Autodesk Inventor part; units mm, degrees
ref_plane "YZ Plane" through (0, 0, 0) normal (1, 0, 0) x (0, 1, 0)
ref_plane "XZ Plane" through (0, 0, 0) normal (0, 1, 0) x (-1, 0, 0)
ref_plane "XY Plane" through (0, 0, 0) normal (0, 0, 1) x (1, 0, 0)
sketch "Sketch1" plane through (0, 0, 0) normal (1, 0, 0) x (0, 1, 0)
  line L0 (15, 25) -> (-5, 25)
  line L1 (-5, 25) -> (-5, -25)
  line L2 (-5, -25) -> (15, -25)
  line L3 (15, -25) -> (0, -10)
  line L4 (0, -10) -> (0, 10)
  line L5 (0, 10) -> (15, 25)
  line L6 (0, 0) -> (-5, 0) construction
  circle A0 centre (5, -20) radius 2
  circle A1 centre (5, 20) radius 2
  dimension "d0" = 50
  dimension "d1" = 45
  dimension "d2" = 5
  dimension "d4" = 40
  dimension "d5" = 4
  dimension "d6" = 20
  dimension "d7" = 5
  dimension "d8" = 15
extrude "Extrusion1" add sketch "Sketch1" along normal blind 5
sketch "Sketch2" plane through (0, 0, 0) normal (-1, 0, 0) x (0, 0, 1)
  line L0 (25, -5) -> (-25, -5)
  line L1 (-25, -5) -> (25, -5)
  line L2 (25, -5) -> (25, 0)
  line L3 (25, 0) -> (-25, 0)
  line L4 (-25, 0) -> (-25, -5)
  point P0 (0, 0)
extrude "Extrusion2" add sketch "Sketch2" along normal blind 10
mirror "Mirror1" about plane through (-10, -2.5, 0) normal (-1, 0, 0)
sketch "Sketch5" plane through (5, -5, -25) normal (0, -1, 0) x (1, 0, 0)
  line L0 (0, 50) -> (0, 0) construction
  line L1 (0, 50) -> (-30, 50)
  line L2 (-30, 50) -> (-30, 55)
  line L3 (-30, 55) -> (0, 55)
  line L4 (0, 55) -> (0, 50)
  line L5 (-30, 0) -> (0, 0)
  line L6 (0, 0) -> (-30, 0)
  line L7 (-30, 0) -> (-30, -5)
  line L8 (-30, -5) -> (0, -5)
  line L9 (0, -5) -> (0, 0)
  line L10 (-30, 50) -> (-30, 0) construction
  point P0 (-5, 25)
  dimension "d19" = 5
extrude "Extrusion5" add sketch "Sketch5" against normal blind 62.5
sketch "Sketch6" plane through (-25, -5, 30) normal (0, 0, 1) x (1, 0, 0)
  line L0 (30, 62.5) -> (25, 62.5)
  line L1 (25, 62.5) -> (25, 47.5)
  line L2 (25, 47.5) -> (30, 47.5)
  line L3 (30, 47.5) -> (30, 62.5)
  line L4 (30, 0) -> (30, 62.5) construction
  dimension "d25" = 5
  dimension "d26" = 15
extrude "Extrusion6" add sketch "Sketch6" along normal blind 60
sketch "Sketch8" plane through (5, 0, 0) normal (1, 0, 0) x (0, 0, -1)
  line L0 (-30, 42.5) -> (-30, 57.5) construction
  line L1 (-30, 50) -> (-90, 50) construction
  line L2 (-90, 42.5) -> (-90, 57.5) construction
  circle A0 centre (-85, 50) radius 2.5
  circle A1 centre (-35, 50) radius 2.5
  point P0 (0, 0)
  dimension "d31" = 5
  dimension "d32" = 5
  dimension "d33" = 5
extrude "Extrusion8" cut sketch "Sketch8" against normal blind 10
mirror "Mirror2" about plane through (0, 0, 0) normal (0, 0, 1) of "Extrusion6", "Extrusion8"
sketch "Sketch7" plane through (-25, -5, 30) normal (0, 0, 1) x (1, 0, 0)
  line L0 (0, 62.5) -> (25, 62.5) construction
  line L1 (0, 0) -> (0, 62.5) construction
  line L2 (0, 62.5) -> (0, 20)
  line L3 (0, 20) -> (0, 62.5)
  line L4 (0, 20) -> (10, 20)
  line L5 (10, 20) -> (20, 30)
  line L6 (0, 20) -> (0, 62.5)
  line L7 (0, 62.5) -> (20, 62.5)
  line L8 (20, 30) -> (20, 62.5)
  line L9 (30, 62.5) -> (0, 62.5) construction
  line L10 (25, 47.5) -> (25, 62.5)
  point P0 (25, 5)
  dimension "d38" = 5
  dimension "d39" = 45
  dimension "d40" = 10
extrude "Extrusion7" cut sketch "Sketch7" along normal through all both and the other way through all
sketch "Sketch3" plane through (0, 0, 10) normal (0, 1, 0) x (1, 0, 0)
  line L0 (-20, 0) -> (-20, -15) construction
  line L1 (0, 20) -> (5, 20) construction
  line L2 (-20, 0) -> (0, 20) construction
  line L3 (-20, 35) -> (-20, 20) construction
  line L4 (0, 0) -> (5, 0) construction
  line L5 (-20, 20) -> (0, 0) construction
  circle A0 centre (-10, 10) radius 3
  point P0 (0, 10)
  dimension "d13" = 6
sketch "Sketch4" plane through (0, 0, 10) normal (0, 1, 0) x (1, 0, 0)
  circle A0 centre (-10, 10) radius 3
  circle A1 centre (-10, 10) radius 2
  point P0 (0, 10)
  dimension "d16" = 4
equation "\"d7\" = 0.333333 * d8"
properties part number "upper fan mount"
Design review of the part built by this model. Coordinates are the model's own, in mm. A direction names the side the tool comes from. Coordinates: 2 decimals unless noted, no trailing zeros. Loops run counter-clockwise (first coordinate to the right, second up) from the corner with the lowest first, then second, coordinate; pieces in that order, holes last.
Q1. To check wall thickness, follow line 1 (Z direction, x = -21, y = 5); line 2 (Y direction, x = 1.4, z = -35); line 3 (Z direction, x = -18.5, y = 2). State the ranges of each line that lie inside material, in increasing order.
Reported:
line 1: z = -30 to -22, -18 to -15, 15 to 18, 22 to 30
line 2: y = 42.5 to 47.5, 52.5 to 57.5
line 3: z = -30 to -25, 25 to 30
Q2. Tool access review of faces 4 (the face through (-5, 22, -25)), 5 (the face through (-20, 15, 27)), 6 (the face through (0, 50, 60)): name each direction out of +Z, -Z, +X, -X, +Y, -Y from which nothing blocks a thin tool from reaching the whole face with its end or side.
Reported:
face 4: +Y
face 5: +Z, -Z, -X, +Y
face 6: +Z, -X, +Y, -Y
Q3. We need section D-D on y = 39.5. State the section outline as (x, z) points, and give its area (3 significant figures).
Reported:
outline: (-5, -30) - (5, -30) - (5, -25) - (-5, -25) - close; (-5, 25) - (5, 25) - (5, 30) - (-5, 30) - close
area: 100 mm2
Q4. We need section C-C on x = 2.5. State the section outline as (y, z) points.
Reported:
outline: (-5, -30) - (42.5, -30) - (42.5, -90) - (57.5, -90) - (57.5, -25) - (15, -25) - (0, -10) - (0, 10) - (15, 25) - (57.5, 25) - (57.5, 90) - (42.5, 90) - (42.5, 30) - (-5, 30) - close; hole circle Ø4 at (5, -20); hole circle Ø4 at (5, 20); hole circle Ø5 at (50, -85); hole circle Ø5 at (50, -35); hole circle Ø5 at (50, 35); hole circle Ø5 at (50, 85)
Q5. We need section A-A on y = 50. State the section outline as (x, z) points, and give its area (3 significant figures).
Reported:
outline: (-5, -30) - (0, -30) - (0, -32.5) - (5, -32.5) - (5, -25) - (-5, -25) - close; (-5, 25) - (5, 25) - (5, 32.5) - (0, 32.5) - (0, 30) - (-5, 30) - close; (0, -90) - (5, -90) - (5, -87.5) - (0, -87.5) - close; (0, -82.5) - (5, -82.5) - (5, -37.5) - (0, -37.5) - close; (0, 37.5) - (5, 37.5) - (5, 82.5) - (0, 82.5) - close; (0, 87.5) - (5, 87.5) - (5, 90) - (0, 90) - close
area: 600 mm2
Q6. The part is to be moulded in two halves that separate along Y. For faces 1 (the face through (0, 4, -22)), 2 (the face through (2, 7, 17)), 3 (the face through (-22.465, 3.526, 21.352)), say which applies: +Y half, -Y half, draft (parallel to the pull), parting line (faces both ways), or undercut.
Reported:
face 1: draft
face 2: +Y half
face 3: undercut
Q7. We need section B-B on z = 20. State the section outline as (x, y) points, and give its area (3 significant figures).
Reported:
outline: (-25, -5) - (5, -5) - (5, 3) - (0, 3) - (0, 0) - (-20, 0) - (-20, 3) - (-25, 3) - close; (-25, 7) - (-20, 7) - (-20, 10) - (-25, 10) - close; (0, 7) - (5, 7) - (5, 10) - (0, 10) - close
area: 210 mm2
Q8. For pin 1 (1.5 mm diameter, centred on x = -19.5, z = 28.5, fed in from +Y); pin 2 (4 mm diameter, centred on x = 1.5, z = -73, fed in from -Y); pin 3 (6 mm diameter, centred on x = -9, y = 36, fed in from -Z); pin 4 (6 mm diameter, centred on x = -6.5, z = 10, fed in from +Y), all flat-tipped, find the tip position at first contact; note any pin that passes through.
Reported:
pin 1: stops at y = 15
pin 2: stops at y = 42.5
pin 3: passes through
pin 4: stops at y = 0
